Can you work these out from the model? Positions are in its coordinate system, mm. Face numbers are marked on the shaded views. A direction names the side the tool comes from. Give positions to 0.01 mm unless a question says otherwise; leave off trailing zeros. Loops run counter-clockwise (first coordinate to the right, second up) from the corner with the lowest first, then second, coordinate; pieces in that order, holes last. Notation, with made-up numbers: (-27, 48) - (8, 48) arc R19 ccw to (8, 79) - close; hole circle Ø8 at (53, 58). An arc over 180 degrees is marked (long way). Answer as a JSON object with one key per item and string values.
```python
from build123d import *

# Parameters (mm, degrees)
F0_W     = 13
F0_H     = 22
F1_DEPTH = 12
F3_DEPTH = 12.001
F5_DEPTH = 9


with BuildPart() as f1:
    # F0 (on Top) → F1 (new body)
    with BuildSketch(Plane.XY):
        with Locations((6.5, -11)):
            Rectangle(F0_W, F0_H)
    extrude(amount=F1_DEPTH)

    # F2 (on face) → F3 (cut, through all)
    with BuildSketch(Plane.XY.offset(12)):
        Polygon((13, -22), (13, -4), (3, -22), align=None)
    extrude(amount=-F3_DEPTH, mode=Mode.SUBTRACT)

    # F4 (on face) → F5 (cut)
    with BuildSketch(Plane.XY.offset(12)):
        Polygon((3, -4), (3, -22), (13, -4), align=None)
    extrude(amount=-F5_DEPTH, mode=Mode.SUBTRACT)


solid = f1.part
```
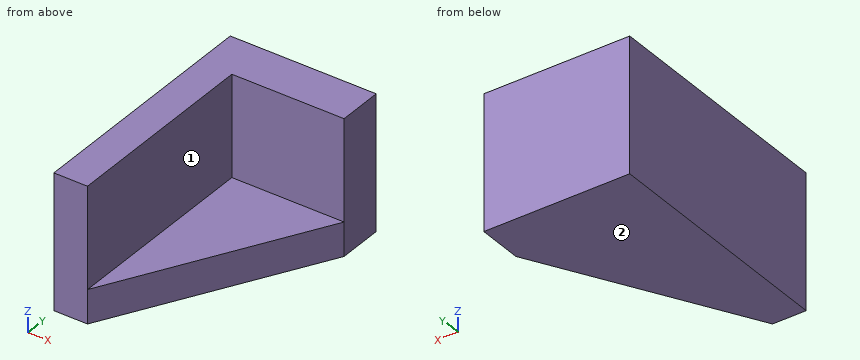
1) Imagine slicing it at B-B on z = 1.25. Write out the boundary of the cut face in (x, y).
Check sheet entries:
{"outline": "(0, -22) - (3, -22) - (13, -4) - (13, 0) - (0, 0) - close"}
2) Which directions (+Z, -Z, +X, -X, +Y, -Y) give clear straight access to the entire face, cutting with the end or side of a thin tool? Please do the marked faces 1 and 2.
Check sheet entries:
{"face 1": "+Z, +X, -Y", "face 2": "-Z, +X, -X, +Y, -Y"}
3) Imagine slicing it at A-A on x = 5. Write out the boundary of the cut face in (y, z), and give its area (3 significant figures).
Check sheet entries:
{"outline": "(-18.4, 0) - (0, 0) - (0, 12) - (-4, 12) - (-4, 3) - (-18.4, 3) - close", "area": "91.2 mm2"}
4) I'm going to push flat-ended pins straight in: P1, Ø2, axis at x = 10.5, z = 2.5, coming from the -Y side; P2, Ø3, axis at x = 6.5, z = 7.5, coming from the -Y side; P3, Ø2, axis at x = 6, y = -8, coming from the +Z side; P4, Ø2, axis at x = 5, z = 9, coming from the +Y side. Where does each tip first touch, or does it pass through?
Check sheet entries:
{"P1": "y = -10.3", "P2": "y = -4", "P3": "z = 3", "P4": "y = 0"}
5) Imagine slicing it at C-C on y = -4.25. Write out the boundary of the cut face in (x, z), and give its area (3 significant figures).
Check sheet entries:
{"outline": "(0, 0) - (12.86, 0) - (12.86, 3) - (3, 3) - (3, 12) - (0, 12) - close", "area": "65.6 mm2"}
6) I need wall thicknesses on L1, parallel to Y at x = 12.25, z = 7; L2, parallel to Z at x = 6, y = -6.25. Which ranges of each line are inside material? Lowest first, please.
Check sheet entries:
{"L1": "-4 to 0", "L2": "0 to 3"}
